Input: part model. Units: mm. Frame: model coordinates. Face numbers are marked on the shaded views. A direction names the side the tool comes from. Give positions to 0.01 mm unless a question says otherwise; leave off trailing zeros. Order: outer loops, then holes, each group sorted by start corner. A loop starts at its lowest first (then second) coordinate and runs counter-clockwise, first axis right, second up. Notation, with made-up numbers: (12.25, -27) - (25.25, -27) arc R18 cw to (25.25, 5) - close; hole circle Ø6 at (27, -9). An arc over 180 degrees is marked (long way). Use a Markdown table: item, result.
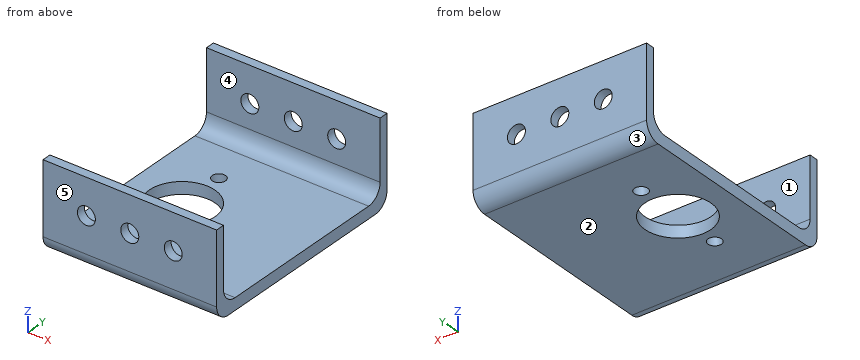
from build123d import *

# Parameters (mm, degrees)
SKETCH3_R           = 11
BOSS_EXTRUDE1_DEPTH = 4
SKETCH5_W           = 58
SKETCH5_H           = 3
BOSS_EXTRUDE2_DEPTH = 25
FILLET1_R           = 5
SKETCH6_R           = 3
CUT_EXTRUDE1_DEPTH  = 89.532479916
SKETCH7_R           = 2.225
CUT_EXTRUDE2_DEPTH  = 62.081912216


with BuildPart() as part:
    # Sketch3 → Boss-Extrude1 (new body)
    with BuildSketch(Plane.XY):
        Polygon((-19, 37), (39, 37), (39, 0), (39, -37), (-19, -37), (-19, 0), align=None)
        with Locations((-1, 0)):
            Circle(SKETCH3_R, mode=Mode.SUBTRACT)
    extrude(amount=BOSS_EXTRUDE1_DEPTH)

    # Sketch5 → Boss-Extrude2 (add)
    with BuildSketch(Plane.XY.offset(4)):
        with Locations((10, 35.5)):
            Rectangle(SKETCH5_W, SKETCH5_H)
        with Locations((10, -35.5)):
            Rectangle(SKETCH5_W, SKETCH5_H)
    extrude(amount=BOSS_EXTRUDE2_DEPTH)

    # Fillet1
    fillet1_edges = [part.edges().sort_by_distance(p)[0] for p in [
        (10, 34, 4),
        (10, -34, 4),
        (10, -37, 0),
        (10, 37, 0),
    ]]
    fillet(fillet1_edges, radius=FILLET1_R)

    # Sketch6 → Cut-Extrude1 (cut, through all)
    with BuildSketch(Plane.XZ.offset(37)):
        with Locations(Location((24.5, 17, 0), (0, 0, 270))):
            Circle(SKETCH6_R)
        with Locations(Location((-4.5, 17, 0), (0, 0, 270))):
            Circle(SKETCH6_R)
        with Locations(Location((10, 17, 0), (0, 0, 270))):
            Circle(SKETCH6_R)
    extrude(amount=-CUT_EXTRUDE1_DEPTH, mode=Mode.SUBTRACT)

    # Sketch7 → Cut-Extrude2 (cut, through all)
    with BuildSketch(Plane(origin=(0, 0, 0), x_dir=(-1, 0, 0), z_dir=(0, 0, -1))):
        with Locations((1, -16)):
            Circle(SKETCH7_R)
        with Locations((1, 16)):
            Circle(SKETCH7_R)
    extrude(amount=-CUT_EXTRUDE2_DEPTH, mode=Mode.SUBTRACT)


solid = part.part
1. Section query C-C (z = 24.25). Return loops of the section in (x, y), then the cut area to 3 significant figures.
Response:
| item | result |
|---|---|
| outline | (-19, -37) - (39, -37) - (39, -34) - (-19, -34) - close; (-19, 34) - (39, 34) - (39, 37) - (-19, 37) - close |
| area | 348 mm^2 |
2. Mould query, pull axis Y, two halves, no side actions, for the marked faces 1, 2 and 3. Classes: pulls with the +Y half, pulls with the -Y half, needs draft (parallel to the pull), parting line crosses it, or undercut.
Response:
| item | result |
|---|---|
| face 1 | undercut |
| face 2 | needs draft |
| face 3 | pulls with the +Y half |
3. Pin query (flat end, axial travel): pin 1 (5 mm diameter, centred on x = -5, y = -29.5, fed in from +Z); pin 2 (9.5 mm diameter, centred on x = 10, z = 17, fed in from +Y). Return the tip coordinate at first contact, or that it passes through.
Response:
| item | result |
|---|---|
| pin 1 | stops at z = 5 |
| pin 2 | stops at y = 37 |
4. Material intervals for line 1 along X through (y, z) = (-35.7, 17); line 2 along Y through (x, z) = (-14.5, 26.5); line 3 along Y through (x, z) = (-1, 2.15) (3 decimals), sorted ascending.
Response:
| item | result |
|---|---|
| line 1 | x = -19 to -7.5, -1.5 to 7, 13 to 21.5, 27.5 to 39 |
| line 2 | y = -37 to -34, 34 to 37 |
| line 3 | y = -36.108 to -18.225, -13.775 to -11, 11 to 13.775, 18.225 to 36.108 |
5. Section query D-D (x = 24.5). Return loops of the section in (y, z), then the cut area to 3 significant figures.
Response:
| item | result |
|---|---|
| outline | (-37, 5) arc R5 ccw to (-32, 0) - (32, 0) arc R5 ccw to (37, 5) - (37, 14) - (34, 14) - (34, 9) arc R5 cw to (29, 4) - (-29, 4) arc R5 cw to (-34, 9) - (-34, 14) - (-37, 14) - close; (-37, 20) - (-34, 20) - (-34, 29) - (-37, 29) - close; (34, 20) - (37, 20) - (37, 29) - (34, 29) - close |
| area | 410 mm^2 |
6. Set-up query: the marked faces 4 and 5. Return all of +Z, -Z, +X, -X, +Y, -Y with unobstructed straight access to the full face (end or side cutting, diameter ignored); none if empty.
Response:
| item | result |
|---|---|
| face 4 | +Z, +X, -X |
| face 5 | +Z, -Z, +X, -X, -Y |
7. Section query B-B (y = 0). Return loops of the section in (x, z), then the cut area to 3 significant figures.
Response:
| item | result |
|---|---|
| outline | (-19, 0) - (-12, 0) - (-12, 4) - (-19, 4) - close; (10, 0) - (39, 0) - (39, 4) - (10, 4) - close |
| area | 144 mm^2 |
8. Section query A-A (z = 17). State how many separate pieces and enclosed holes the cut face has, then the cut area to 3 significant figures.
Response:
| item | result |
|---|---|
| separate pieces | 8 |
| enclosed holes | 0 |
| area | 240 mm^2 |
